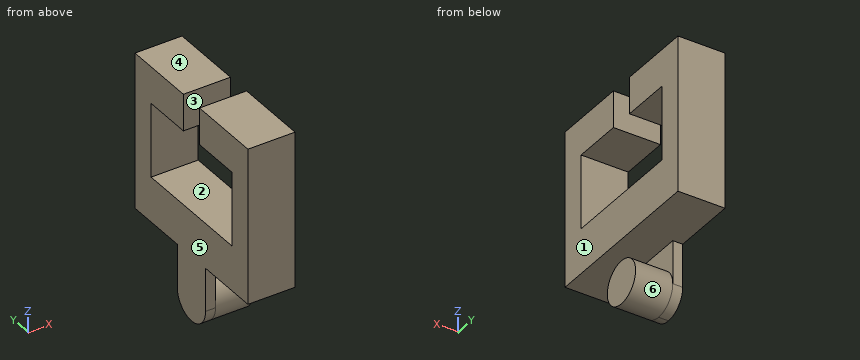
from build123d import *

# Parameters (mm, degrees)
SKETCH1_R           = 11.112754
BOSS_EXTRUDE1_DEPTH = 9.525
SKETCH2_W           = 22.225508
SKETCH2_H           = 33.338262
BOSS_EXTRUDE2_DEPTH = 5.091684
FILLET1_R           = 11.112754
FILLET2_R           = 11.112754
SKETCH1_3_W         = 12.6492
SKETCH1_3_H         = 38.0746
BOSS_EXTRUDE3_DEPTH = 9.525
BOSS_EXTRUDE6_DEPTH = 5.091684


with BuildPart() as part:
    # Sketch1 → Boss-Extrude1 (new, symmetric)
    with BuildSketch(Plane.YZ):
        with Locations(Location((0, -22.225508, 0), (0, 0, 90))):
            Circle(SKETCH1_R)
    extrude(amount=BOSS_EXTRUDE1_DEPTH, both=True)

    # Sketch2 → Boss-Extrude2 (add)
    with BuildSketch(Plane(origin=(-9.525, 0, 0), x_dir=(0, -1, 0), z_dir=(-1, 0, 0))):
        with Locations((0, -16.669131)):
            Rectangle(SKETCH2_W, SKETCH2_H)
    extrude(amount=BOSS_EXTRUDE2_DEPTH)

    # Fillet1
    fillet1_edges = [part.edges().sort_by_distance(p)[0] for p in [
        (-12.070842, 11.112754, -33.338262),
    ]]
    fillet(fillet1_edges, radius=FILLET1_R)

    # Fillet2
    fillet2_edges = [part.edges().sort_by_distance(p)[0] for p in [
        (-12.070842, -11.112754, -33.338262),
    ]]
    fillet(fillet2_edges, radius=FILLET2_R - 0.0001)  # a hair under: the kernel refuses the full size



with BuildPart() as body_2:
    # Sketch1<3> → Boss-Extrude3 (new, symmetric)
    with BuildSketch(Plane.YZ):
        with Locations((-38.02888, 42.162476)):
            Rectangle(SKETCH1_3_W, SKETCH1_3_H)
        Polygon((-31.70428, 23.125176), (-44.35348, 23.125176), (-44.35348, 0), (44.35348, 0), (44.35348, 23.125176), (31.70428, 23.125176), align=None)
        Polygon((-44.35348, 80.091534), (-44.35348, 61.199776), (-31.70428, 61.199776), (-6.3246, 61.199776), (-6.3246, 80.091534), align=None)
        with Locations((38.02888, 42.162476)):
            Rectangle(SKETCH1_3_W, SKETCH1_3_H)
        Polygon((6.3246, 61.199776), (31.70428, 61.199776), (44.35348, 61.199776), (44.35348, 80.091534), (6.3246, 80.091534), align=None)
    extrude(amount=BOSS_EXTRUDE3_DEPTH, both=True)


with BuildPart() as part_1:
    add(part.part)

    add(body_2.part)  # Boss-Extrude6 merges body 2
    # Sketch8 → Boss-Extrude6 (add)
    with BuildSketch(Plane(origin=(-9.525, 0, 0), x_dir=(0, -1, 0), z_dir=(-1, 0, 0))):
        Polygon((31.70428, 61.199776), (31.70428, 23.125176), (-31.70428, 23.125176), (-31.70428, 61.199776), (-6.3246, 61.199776), (-6.3246, 80.091534), (-44.35348, 80.091534), (-44.35348, 0), (44.35348, 0), (44.35348, 80.091534), (6.3246, 80.091534), (6.3246, 61.199776), align=None)
    extrude(amount=BOSS_EXTRUDE6_DEPTH)


solid = part_1.part
Design review of the part built by this model. Coordinates are the model's own, in mm. Face numbers are marked on the shaded views. A direction names the side the tool comes from. Give positions to 0.01 mm unless a question says otherwise; leave off trailing zeros. Loops run counter-clockwise (first coordinate to the right, second up) from the corner with the lowest first, then second, coordinate; pieces in that order, holes last. Notation, with made-up numbers: (-28.75, 35.5) -> (23.25, 35.5) arc R24 ccw to (23.25, 65.5) -> close; hole circle Ø7 at (1, 74.25). An arc over 180 degrees is marked (long way). One line per question, with ' | ' between items. Start each with the question number.
(1) For line 1 (Y direction, x = -5.5, z = 75.5); line 2 (Z direction, x = 5.25, y = 9.5); line 3 (Y direction, x = -6.5, z = 53.5), list the stretches that pass through material, from the lowest coordinate up.
(2) Draft analysis for pull direction Z (two halves, no side actions). For the marked faces 4, 5 and 6, state which applies: +Z half, -Z half, draft (parallel to the pull), parting line (faces both ways), or undercut.
(3) We need section B-B (x = 8). State the section outline as (y, z) points.
(4) We need section A-A (y = -20). State the section outline as (x, z) points (3 decimals), and give its area (3 significant figures).
(5) We need section C-C (z = 68). State the section outline as (x, y) points (3 decimals), and give its area (3 significant figures).
(6) For the marked faces 1, 2 and 3, list the 3-axis set-ups (+Z, -Z, +X, -X, +Y, -Y) from which the entire face can be reached by the end or side of a thin tool; tool diameter is ignored.
(7) Insertion check: P1, Ø2, axis at x = 0.5, z = -12.5, coming from the -Y side; P2, Ø1.5, axis at x = -11.5, z = -9, coming from the -Y side; P3, Ø10, axis at x = 0, z = -7, coming from the -Y side. Each pin has a flat end and moves straight along its axis. Give the tip position at first contact, or say it passes through.
The answers:
1) line 1: y = -44.35 to -6.32, 6.32 to 44.35 | line 2: z = -27.99 to -16.46, 0 to 23.13, 61.2 to 80.09 | line 3: y = -44.35 to -31.7, 31.7 to 44.35
2) face 4: +Z half | face 5: draft | face 6: undercut
3) outline: (-44.35, 0) -> (44.35, 0) -> (44.35, 80.09) -> (6.32, 80.09) -> (6.32, 61.2) -> (31.7, 61.2) -> (31.7, 23.13) -> (-31.7, 23.13) -> (-31.7, 61.2) -> (-6.32, 61.2) -> (-6.32, 80.09) -> (-44.35, 80.09) -> close; circle Ø22.23 at (0, -22.23)
4) outline: (-14.617, 0) -> (9.525, 0) -> (9.525, 23.125) -> (-14.617, 23.125) -> close; (-14.617, 61.2) -> (9.525, 61.2) -> (9.525, 80.092) -> (-14.617, 80.092) -> close | area: 1,010 mm^2
5) outline: (-14.617, -44.353) -> (9.525, -44.353) -> (9.525, -6.325) -> (-14.617, -6.325) -> close; (-14.617, 6.325) -> (9.525, 6.325) -> (9.525, 44.353) -> (-14.617, 44.353) -> close | area: 1,840 mm^2
6) face 1: +Z, -Z, +X, +Y, -Y | face 2: +X, -X | face 3: +Z, +X, -X
7) P1: stops at y = -6.88 | P2: stops at y = -11.11 | P3: stops at y = -4.35
